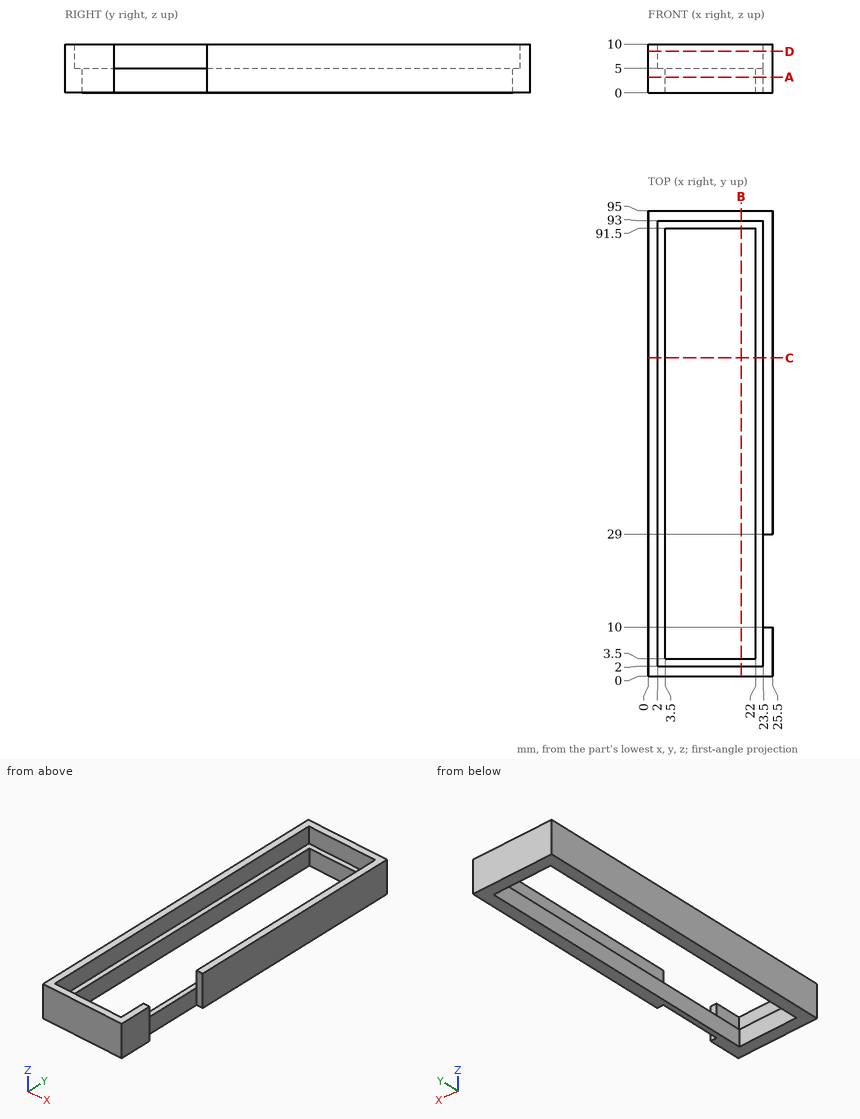
Answer from the drawing. Dimensions are ordinates in mm from the lowest x, y and z of the part. Coordinates: 2 decimals unless noted, no trailing zeros. Order: outer loops, then holes, each group sorted by start corner. A loop starts at its lowest first (then second) coordinate and runs counter-clockwise, first axis right, second up. Notation, with made-up numbers: (15.5, -6.75) - (19.5, -6.75) arc R15 cw to (19.5, 8.25) - close; hole circle Ø4 at (65, -13.5). An arc over 180 degrees is marked (long way). Put each result on its own line as item: value. Start each with the question number.
1) Find the intervals of material crossed by line 1 (Y direction, x = 8.5, z = 5.5); line 2 (X direction, y = 40, z = 1.25); line 3 (Y direction, x = 5, z = 3.75), in increasing order. Write a range as from..to.
2) Find section C-C (y = 65). Give the vertices of the cut face in (x, z), plus the area to 3 significant figures.
3) Find section A-A (z = 3.25). Give the vertices of the cut face in (x, y), plus the area to 4 significant figures.
4) Find section B-B (x = 19). Give the vertices of the cut face in (y, z).
5) Find section D-D (z = 8.5). Give the vertices of the cut face in (x, y).
6) A flat-ended cylindrical pin translates along its axis: pin 1 (2.5 mm diameter, centred on y = 18.5, z = 2.5, fed in from +X). Find the tip coordinate at first contact, or state that the pin passes through.
Results list:
1. line 1: y = 0..2, 93..95
1. line 2: x = 0..3.5, 22..25.5
1. line 3: y = 0..3.5, 91.5..95
2. outline: (0, 0) - (3.5, 0) - (3.5, 5) - (2, 5) - (2, 10) - (0, 10) - close; (22, 0) - (25.5, 0) - (25.5, 10) - (23.5, 10) - (23.5, 5) - (22, 5) - close
2. area: 55.0 mm^2
3. outline: (0, 0) - (25.5, 0) - (25.5, 10) - (23.5, 10) - (23.5, 29) - (25.5, 29) - (25.5, 95) - (0, 95) - close; hole (3.5, 3.5) - (22, 3.5) - (22, 91.5) - (3.5, 91.5) - close
3. area: 756.5 mm^2
4. outline: (0, 0) - (3.5, 0) - (3.5, 5) - (2, 5) - (2, 10) - (0, 10) - close; (91.5, 0) - (95, 0) - (95, 10) - (93, 10) - (93, 5) - (91.5, 5) - close
5. outline: (0, 0) - (25.5, 0) - (25.5, 10) - (23.5, 10) - (23.5, 2) - (2, 2) - (2, 93) - (23.5, 93) - (23.5, 29) - (25.5, 29) - (25.5, 95) - (0, 95) - close
6. pin 1: stops at x = 23.5
